Model file for the job. Use its own axes, mm. A direction names the side the tool comes from. Round coordinates to 2 decimals unless told otherwise and drop trailing zeros. Order: outer loops, then holes, each group sorted by start corner. A loop starts at its lowest first (then second) coordinate and runs counter-clockwise, first axis right, second up. Notation, with made-up numbers: M 10.5,-17 L 60.5,-17 A9 ccw 60.5,-9 Z; hole C 73,50 d4. An arc over 180 degrees is marked long. Return JSON: item names as keys, results as strings. Group by question number.
Item 1: Probe line 1 along Y through (x, z) = (0, 1.95); line 2 along X through (y, z) = (-2, 1.45); line 3 along Y through (x, z) = (7, 1.6). List the from-to ranges inside material, lowest first.
Item 2: Pin check, flat tips, straight feed: pin 1 Ø4 at (x, y) = (-35, 0) entering from +Z; pin 2 Ø1 at (x, z) = (-6.5, 2) entering from +Y; pin 3 Ø0.9 at (y, z) = (-24.5, 2) entering from -X; pin 4 Ø0.9 at (y, z) = (-29, 1.5) entering from +X. Stop position of each tip, or through.
Item 3: Slice it at B-B on x = 1. Write the cut outline in (y, z), then the cut area to 3 significant figures.
Item 4: Which spindle directions (+Z, -Z, +X, -X, +Y, -Y) get a long thin tool onto all of the face, cutting with end or side? Do faces 1 (the face through (5, 24, 2)), 2 (the face through (10, 0, 1)), 3 (the face through (-5, -21, 1)). Say none if no direction does.
Item 5: Slice it at D-D on x = -7. Write the cut outline in (y, z).
Item 6: Slice it at C-C on y = -23. Write the cut outline in (x, z).
Item 7: Pull direction X, two halves, no side cores. Call faces 4 (the face through (5, -24, 2)), 5 (the face through (5.35, 0.07, 1.48)), 6 (the face through (-9.8, 0.6, 3)): pulls with the +X half, pulls with the -X half, needs draft (parallel to the pull), parting line crosses it, or undercut.
Item 8: Slice it at A-A on z = 1.7. Write the cut outline in (x, y).
from build123d import *

# Parameters (mm, degrees)
SKETCH1_R           = 40
SKETCH1_R_2         = 3
SKETCH1_R_3         = 1.65
SKETCH1_R_4         = 2.2
BOSS_EXTRUDE1_DEPTH = 3
CUT_EXTRUDE1_DEPTH  = 10


with BuildPart() as part:
    # Sketch1 → Boss-Extrude1 (new body)
    with BuildSketch(Plane.XY):
        Circle(SKETCH1_R)
        with BuildLine():
            Line((5, -34.641016151), (5, -8.660254038))
            ThreePointArc((5, -8.660254038), (10, 0), (5, 8.660254038))
            Line((5, 8.660254038), (5, 34.641016151))
            ThreePointArc((5, 34.641016151), (35, 0), (5, -34.641016151))
        make_face(mode=Mode.SUBTRACT)
        with BuildLine():
            Line((-5, 34.641016151), (-5, 8.660254038))
            ThreePointArc((-5, 8.660254038), (-10, 0), (-5, -8.660254038))
            Line((-5, -8.660254038), (-5, -34.641016151))
            ThreePointArc((-5, -34.641016151), (-24.753298969, -24.744174873), (-34.642857143, -4.987228587))
            ThreePointArc((-34.642857143, -4.987228587), (-30, 0), (-34.642857143, 4.987228587))
            ThreePointArc((-34.642857143, 4.987228587), (-24.753298969, 24.744174873), (-5, 34.641016151))
        make_face(mode=Mode.SUBTRACT)
        Circle(SKETCH1_R_2, mode=Mode.SUBTRACT)
        with Locations((-7, 0)):
            Circle(SKETCH1_R_3, mode=Mode.SUBTRACT)
        with Locations((7, 0)):
            Circle(SKETCH1_R_3, mode=Mode.SUBTRACT)
        with Locations((-35, 0)):
            Circle(SKETCH1_R_4, mode=Mode.SUBTRACT)
    extrude(amount=BOSS_EXTRUDE1_DEPTH)

    # Sketch3 → Cut-Extrude1 (cut)
    with BuildSketch(Plane.XY.offset(3)):
        Polygon((5, 39.686269666), (5, 8.660254038), (14.289111203, 8.660254038), (14.289111203, -8.660254038), (5, -8.660254038), (5, -39.686269666), (45, -39.686269666), (45, 39.686269666), align=None)
    extrude(amount=-CUT_EXTRUDE1_DEPTH, mode=Mode.SUBTRACT)


solid = part.part
Output values:
{
 "1": {"line 1": "-40 to -3, 3 to 40", "line 2": "-39.95 to -35.92, -34.08 to -30.42, -9.8 to -2.24, 2.24 to 9.8", "line 3": "-7.14 to -1.65, 1.65 to 7.14"},
 "2": {"pin 1": "through", "pin 2": "y = 39.55", "pin 3": "x = -31.96", "pin 4": "x = 5"},
 "3": {"outline": "M -39.99,0 L -2.83,0 L -2.83,3 L -39.99,3 Z; M 2.83,0 L 39.99,0 L 39.99,3 L 2.83,3 Z", "area": "223 mm²"},
 "4": {"face 1": "+Z, -Z, +X, +Y", "face 2": "+Z, -Z, +X", "face 3": "+Z, -Z"},
 "5": {"outline": "M -39.38,0 L -34.29,0 L -34.29,3 L -39.38,3 Z; M -7.14,0 L -1.65,0 L -1.65,3 L -7.14,3 Z; M 1.65,0 L 7.14,0 L 7.14,3 L 1.65,3 Z; M 34.29,0 L 39.38,0 L 39.38,3 L 34.29,3 Z"},
 "6": {"outline": "M -32.73,0 L -26.38,0 L -26.38,3 L -32.73,3 Z; M -5,0 L 5,0 L 5,3 L -5,3 Z"},
 "7": {"face 4": "pulls with the +X half", "face 5": "undercut", "face 6": "needs draft"},
 "8": {"outline": "M 5,-39.69 L 5,-8.66 A10 ccw 5,8.66 L 5,39.69 A40 ccw long Z; hole C -35,0 d4.4; hole M -34.64,-4.99 A35 ccw -5,-34.64 L -5,-8.66 A10 cw -5,8.66 L -5,34.64 A35 ccw -34.64,4.99 A5 cw Z; hole C -7,0 d3.3; hole C 0,0 d6; hole C 7,0 d3.3"}
}
